Model file for the job. Use its own axes, mm. Face numbers are marked on the shaded views. Coordinates: 2 decimals unless noted, no trailing zeros. Loops run counter-clockwise (first coordinate to the right, second up) from the corner with the lowest first, then second, coordinate; pieces in that order, holes last. Notation, with made-up numbers: (80.25, 18) -> (90.25, 18) arc R11 cw to (90.25, 29) -> close; hole circle Ø8 at (78, -36). An arc over 180 degrees is marked (long way). Use one line per item in the form item = value.
```python
from build123d import *

# Parameters (mm, degrees)
BOSS_EXTRUDE1_DEPTH = 6.35
SKETCH1_3_R         = 12.7
BOSS_EXTRUDE2_DEPTH = 19.05
BOSS_EXTRUDE3_START = 12.7
BOSS_EXTRUDE3_DEPTH = 12.7


with BuildPart() as part:
    # Sketch1 → Boss-Extrude1 (new body)
    with BuildSketch(Plane(origin=(0, 0, 0), x_dir=(1, 0, 0), z_dir=(0, 1, 0))):
        with BuildLine():
            Line((76.2, 4.7625), (11.773215098, 4.7625))
            ThreePointArc((11.773215098, 4.7625), (12.466150804, 2.425919233), (12.7, 0))
            ThreePointArc((12.7, 0), (12.466150804, -2.425919233), (11.773215098, -4.7625))
            Line((11.773215098, -4.7625), (76.2, -4.7625))
            ThreePointArc((76.2, -4.7625), (71.4375, 0), (76.2, 4.7625))
        make_face()
        with BuildLine():
            ThreePointArc((80.9625, 0), (79.567596045, 3.367596045), (76.2, 4.7625))
            Line((76.2, 4.7625), (76.2, -4.7625))
            ThreePointArc((76.2, -4.7625), (79.567596045, -3.367596045), (80.9625, 0))
        make_face()
        with BuildLine():
            Line((76.2, -4.7625), (76.2, 4.7625))
            ThreePointArc((76.2, 4.7625), (71.4375, 0), (76.2, -4.7625))
        make_face()
    extrude(amount=-BOSS_EXTRUDE1_DEPTH)

    # Sketch1_3 → Boss-Extrude2 (add)
    with BuildSketch(Plane(origin=(0, 0, 0), x_dir=(1, 0, 0), z_dir=(0, 1, 0))):
        with Locations(Location((0, 0, 0), (0, 0, 270))):
            Circle(SKETCH1_3_R)
        with BuildLine():
            ThreePointArc((6.35, -4.7625), (-7.9375, 0), (6.35, 4.7625))
            Line((6.35, 4.7625), (6.35, -4.7625))
        make_face(mode=Mode.SUBTRACT)
    extrude(amount=-BOSS_EXTRUDE2_DEPTH)

    # Sketch1_4 → Boss-Extrude3 (add)
    with BuildSketch(Plane(origin=(0, 0, 0), x_dir=(1, 0, 0), z_dir=(0, 1, 0)).offset(BOSS_EXTRUDE3_START)):
        with BuildLine():
            ThreePointArc((80.9625, 0), (79.567596045, 3.367596045), (76.2, 4.7625))
            Line((76.2, 4.7625), (76.2, -4.7625))
            ThreePointArc((76.2, -4.7625), (79.567596045, -3.367596045), (80.9625, 0))
        make_face()
        with BuildLine():
            Line((76.2, -4.7625), (76.2, 4.7625))
            ThreePointArc((76.2, 4.7625), (71.4375, 0), (76.2, -4.7625))
        make_face()
    extrude(amount=-BOSS_EXTRUDE3_DEPTH)


solid = part.part
```
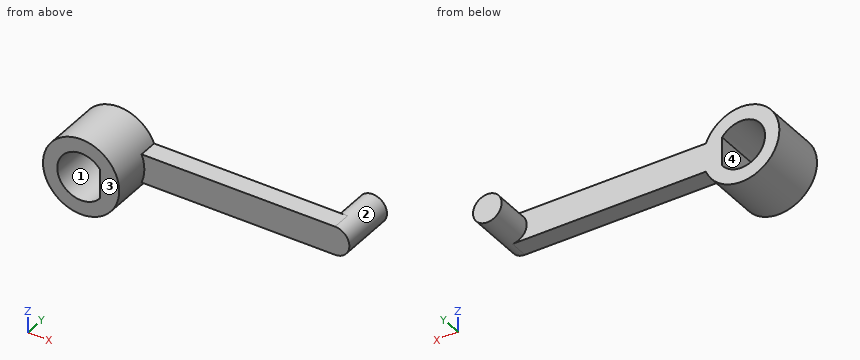
Q1. Pin check, flat tips, straight feed: pin 1 Ø2 at (y, z) = (2.5, -1) entering from -X; pin 2 Ø1 at (x, z) = (49.5, 1) entering from -Y; pin 3 Ø4 at (x, y) = (37.5, -1.5) entering from +Z. Stop position of each tip, or through.
Result:
pin_1 = 71.44
pin_2 = -6.35
pin_3 = 4.76
Q2. Band-saw the part on A-A, the plane x = 3. Write the cut outline in (y, z), and give its area (3 significant figures).
Result:
outline = (-19.05, -12.34) -> (0, -12.34) -> (0, -7.35) -> (-19.05, -7.35) -> close; (-19.05, 7.35) -> (0, 7.35) -> (0, 12.34) -> (-19.05, 12.34) -> close
area = 190 mm2
Q3. Band-saw the part on B-B, the plane z = 7. Write the cut outline in (x, y), and give its area (3 significant figures).
Result:
outline = (-10.6, -19.05) -> (-3.74, -19.05) -> (-3.74, 0) -> (-10.6, 0) -> close; (3.74, -19.05) -> (10.6, -19.05) -> (10.6, 0) -> (3.74, 0) -> close
area = 261 mm2
Q4. Wall check: line 1 along X through (y, z) = (-7.25, 0); line 2 along X through (y, z) = (-3.75, 0); line 3 along Z through (x, y) = (0, -14). Give the ranges that are in metal, low to high.
Result:
line_1 = -12.7 to -7.94, 6.35 to 12.7
line_2 = -12.7 to -7.94, 6.35 to 80.96
line_3 = -12.7 to -7.94, 7.94 to 12.7
Q5. Band-saw the part on D-D, the plane z = 0. Write the cut outline in (x, y).
Result:
outline = (-12.7, -19.05) -> (-7.94, -19.05) -> (-7.94, 0) -> (-12.7, 0) -> close; (6.35, -19.05) -> (12.7, -19.05) -> (12.7, -6.35) -> (80.96, -6.35) -> (80.96, 12.7) -> (71.44, 12.7) -> (71.44, 0) -> (6.35, 0) -> close
Q6. Mould opens along X. For the marked faces 1, 2, 3 and 4 say: released by +X, released by -X, zero draft, split by the parting line, or undercut.
Result:
face_1 = undercut
face_2 = split by the parting line
face_3 = zero draft
face_4 = undercut
